from build123d import *

# Parameters (mm, degrees)
BOSS_EXTRUDE1_DEPTH = 71.5
BOSS_EXTRUDE2_DEPTH = 0.5
BOSS_EXTRUDE3_DEPTH = 0.5


with BuildPart() as part:
    # Sketch1 → Boss-Extrude1 (new, symmetric)
    with BuildSketch(Plane.XY):
        with BuildLine():
            Line((0, 0), (0, 15.5))
            ThreePointArc((0, 15.5), (3.121859218, 20.133852307), (8.589034881, 18.981210799))
            Line((8.589034881, 18.981210799), (13.864340006, 13.54251283))
            ThreePointArc((13.864340006, 13.54251283), (14.078923552, 13.207723175), (14.146067988, 12.81577696))
            Line((14.146067988, 12.81577696), (14.140269037, 12.625696624))
            ThreePointArc((14.140269037, 12.625696624), (14.207413473, 12.233750409), (14.421997019, 11.898960755))
            Line((14.421997019, 11.898960755), (20.098912151, 6.04621365))
            ThreePointArc((20.098912151, 6.04621365), (20.427002666, 5.821520915), (20.816719127, 5.742455809))
            Line((20.816719127, 5.742455809), (21.006887899, 5.742455809))
            ThreePointArc((21.006887899, 5.742455809), (21.39660436, 5.663390704), (21.724694875, 5.438697969))
            Line((21.724694875, 5.438697969), (27, 0))
            Line((27, 0), (26.641096512, -0.34812108))
            Line((26.641096512, -0.34812108), (21.365791387, 5.090576889))
            ThreePointArc((21.365791387, 5.090576889), (21.20174613, 5.202923257), (21.006887899, 5.242455809))
            Line((21.006887899, 5.242455809), (20.816719127, 5.242455809))
            ThreePointArc((20.816719127, 5.242455809), (20.232144435, 5.361053468), (19.740008663, 5.69809257))
            Line((19.740008663, 5.69809257), (14.063093531, 11.550839675))
            ThreePointArc((14.063093531, 11.550839675), (13.741218212, 12.053024156), (13.640501557, 12.640943479))
            Line((13.640501557, 12.640943479), (13.646300509, 12.831023815))
            ThreePointArc((13.646300509, 12.831023815), (13.612728291, 13.026996922), (13.505436518, 13.19439175))
            Line((13.505436518, 13.19439175), (8.230131393, 18.633089719))
            ThreePointArc((8.230131393, 18.633089719), (3.309673296, 19.670467076), (0.5, 15.5))
            Line((0.5, 15.5), (0.5, 0))
            Line((0.5, 0), (0, 0))
        make_face()
    extrude(amount=BOSS_EXTRUDE1_DEPTH, both=True)

    # Sketch2 → Boss-Extrude2 (add)
    with BuildSketch(Plane(origin=(0, 0, 0), x_dir=(0, 0, -1), z_dir=(1, 0, 0))):
        with BuildLine():
            Line((-71.5, 0), (-75, 0))
            ThreePointArc((-75, 0), (-75.707106781, 0.292893219), (-76, 1))
            Line((-76, 1), (-76, 7))
            ThreePointArc((-76, 7), (-75.707106781, 7.707106781), (-75, 8))
            Line((-75, 8), (-71.5, 8))
            Line((-71.5, 8), (-71.5, 0))
        make_face()
        with BuildLine():
            Line((71.5, 8), (71.5, 0))
            Line((71.5, 0), (75, 0))
            ThreePointArc((75, 0), (75.707106781, 0.292893219), (76, 1))
            Line((76, 1), (76, 7))
            ThreePointArc((76, 7), (75.707106781, 7.707106781), (75, 8))
            Line((75, 8), (71.5, 8))
        make_face()
    extrude(amount=BOSS_EXTRUDE2_DEPTH)

    # Sketch3 → Boss-Extrude3 (add)
    with BuildSketch(Plane(origin=(13.911665086, 13.493721942, 0), x_dir=(0, 0, -1), z_dir=(0.7178069761649953, 0.696242159718058, 0))):
        with BuildLine():
            Line((-71.5, -11.221713136), (-75, -11.221713136))
            ThreePointArc((-75, -11.221713136), (-75.707106781, -11.514606354), (-76, -12.221713136))
            Line((-76, -12.221713136), (-76, -17.798538312))
            ThreePointArc((-76, -17.798538312), (-75.707106781, -18.505645094), (-75, -18.798538312))
            Line((-75, -18.798538312), (-71.5, -18.798538312))
            Line((-71.5, -18.798538312), (-71.5, -11.221713136))
        make_face()
        with BuildLine():
            Line((71.5, -18.798538312), (71.5, -11.221713136))
            Line((71.5, -11.221713136), (75, -11.221713136))
            ThreePointArc((75, -11.221713136), (75.707106781, -11.514606354), (76, -12.221713136))
            Line((76, -12.221713136), (76, -17.798538312))
            ThreePointArc((76, -17.798538312), (75.707106781, -18.505645094), (75, -18.798538312))
            Line((75, -18.798538312), (71.5, -18.798538312))
        make_face()
    extrude(amount=-BOSS_EXTRUDE3_DEPTH)


solid = part.part
The listing builds one solid part. Answer for the finished solid, in the listing's coordinates (mm). A direction names the side the tool comes from. Coordinates: 2 decimals unless noted, no trailing zeros. Loops run counter-clockwise (first coordinate to the right, second up) from the corner with the lowest first, then second, coordinate; pieces in that order, holes last.
1) Flat-ended cylindrical pins translate along their axes: pin 1 Ø2 at (x, y) = (20, 6) entering from +Z; pin 2 Ø6 at (x, z) = (21.5, 18) entering from -Y; pin 3 Ø2 at (x, z) = (18, 9.5) entering from +Y; pin 4 Ø10 at (y, z) = (5, -48) entering from -X. Find the tip coordinate at first contact, or state that the pin passes through.
2) Find section D-D on x = 10.75. Write down the section's boundary in (y, z), then the cut area to 3 significant figures.
3) Determine the mould class of faces 1 (the face through (3.38, 19.7, 1)), 2 (the face through (17.221, 9.014, 1.001)), 3 (the face through (10.9, 15.88, 1)), 4 (the face through (0, 8, -1)) for opening direction X: pulls with the +X half, pulls with the -X half, needs draft (parallel to the pull), parting line crosses it, or undercut.
4) Find section A-A on y = 9.5. Write down the section's boundary in (x, z).
5) Find the intervals of material crossed by L1, parallel to X at y = 18.5, z = -39; L2, parallel to X at y = 7, z = -29.5; L3, parallel to Y at x = 4.75, z = -65.5, in increasing order.
6) Find section B-B on z = 2. Write down the section's boundary in (x, y).
7) A tool of negligible diameter and unlimited length cuts with its end or side. For faces 5 (the face through (11.19, 16.3, 1)), 6 (the face through (16.941, 8.583, 1.001)), from which of +Z, -Z, +X, -X, +Y, -Y can it reach the whole face along a straight path? Write none if from no direction.
8) Find section C-C on x = 2.5. Write down the section's boundary in (y, z).
Values:
1. pin 1: stops at z = 71.5
1. pin 2: stops at y = 1.86
1. pin 3: stops at y = 9.24
1. pin 4: stops at x = 0
2. outline: (16.04, -71.5) - (16.75, -71.5) - (16.75, 71.5) - (16.04, 71.5) - close
2. area: 103 mm2
3. face 1: undercut
3. face 2: pulls with the +X half
3. face 3: undercut
3. face 4: pulls with the -X half
4. outline: (0, -71.5) - (0.5, -71.5) - (0.5, 71.5) - (0, 71.5) - close; (16.05, -71.5) - (16.75, -71.5) - (16.75, 71.5) - (16.05, 71.5) - close
5. L1: x = 1 to 1.65, 8.36 to 9.06
5. L2: x = 0 to 0.5, 18.48 to 19.17
5. L3: y = 19.99 to 20.49
6. outline: (0, 0) - (0.5, 0) - (0.5, 15.5) arc R4.5 cw to (8.23, 18.63) - (13.51, 13.19) arc R0.5 cw to (13.65, 12.83) - (13.64, 12.64) arc R1.5 ccw to (14.06, 11.55) - (19.74, 5.7) arc R1.5 ccw to (20.82, 5.24) - (21.01, 5.24) arc R0.5 cw to (21.37, 5.09) - (26.64, -0.35) - (27, 0) - (21.72, 5.44) arc R1 ccw to (21.01, 5.74) - (20.82, 5.74) arc R1 cw to (20.1, 6.05) - (14.42, 11.9) arc R1 cw to (14.14, 12.63) - (14.15, 12.82) arc R1 ccw to (13.86, 13.54) - (8.59, 18.98) arc R5 ccw to (0, 15.5) - close
7. face 5: +Z, -Z, +X, +Y
7. face 6: +Z, -Z, -Y
8. outline: (19.24, -71.5) - (19.83, -71.5) - (19.83, 71.5) - (19.24, 71.5) - close
